The listing builds one solid part. Answer for the finished solid, in the listing's coordinates (mm). Give positions to 0.01 mm unless a question says otherwise; leave off trailing zeros. Loops run counter-clockwise (first coordinate to the right, second up) from the corner with the lowest first, then second, coordinate; pieces in that order, holes last. Notation, with made-up numbers: (8, -4) - (62, -4) arc R29 ccw to (62, 23) - close; hole circle Ø7 at (-11, -35). An arc over 180 degrees is marked (long way). Write each question's results on one line, items separated by ' | '.
from build123d import *

# Parameters (mm, degrees)
SKETCH4_R           = 4.5
BOSS_EXTRUDE1_DEPTH = 4.5
SKETCH5_OUTSIDE_W   = 56.268
SKETCH5_OUTSIDE_H   = 53.856
SKETCH5_OUTSIDE_R   = 7.794228634
CUT_EXTRUDE1_DEPTH  = 9
CUT_EXTRUDE1_TAPER  = 60


with BuildPart() as part:
    # Sketch4 → Boss-Extrude1 (new body, symmetric)
    with BuildSketch(Plane.XY):
        Polygon((4.5, 7.794228634), (-4.5, 7.794228634), (-9, 0), (-4.5, -7.794228634), (4.5, -7.794228634), (9, 0), align=None)
        Circle(SKETCH4_R, mode=Mode.SUBTRACT)
    extrude(amount=BOSS_EXTRUDE1_DEPTH, both=True)

    # Sketch5 outside → Cut-Extrude1 (cut)
    with BuildSketch(Plane.XY.offset(4.5)):
        Rectangle(SKETCH5_OUTSIDE_W, SKETCH5_OUTSIDE_H)
        Circle(SKETCH5_OUTSIDE_R, mode=Mode.SUBTRACT)
    cut_extrude1 = extrude(amount=-CUT_EXTRUDE1_DEPTH, taper=CUT_EXTRUDE1_TAPER, mode=Mode.SUBTRACT)

    # Mirror1: Cut-Extrude1 across plane
    add(cut_extrude1.mirror(Plane.XY), mode=Mode.SUBTRACT)


solid = part.part
Item 1: A flat-ended cylindrical pin translates along its axis: P1, Ø1.5, axis at y = -1.5, z = 2.5, coming from the +X side. Find the tip coordinate at first contact, or state that the pin passes through.
Values found:
P1: stops at x = 8.57
Item 2: Find the intervals of material crossed by line 1 along Y through (x, z) = (0, 1); line 2 along X through (y, z) = (2.75, -0.25); line 3 along X through (y, z) = (-3.75, 0), in increasing order. Write a range as [from, to].
Values found:
line 1: y = [-7.79, -4.5], [4.5, 7.79] | line 2: x = [-7.41, -3.56], [3.56, 7.41] | line 3: x = [-6.83, -2.49], [2.49, 6.83]
Item 3: A cutting plane is placed at A-A, the plane z = -2.5. Determine the outline of the cut face in (x, y).
Values found:
outline: (-9, 0) - (-4.5, -7.79) - (4.5, -7.79) - (9, 0) - (4.5, 7.79) - (-4.5, 7.79) - close; hole circle Ø9 at (0, 0)
Item 4: For a pull along X with two mould halves and no side action, classify faces 1 (the face through (6.781, 3.843, 0.063)), 2 (the face through (-0.59, 4.46, -0.06)), 3 (the face through (-8.09, -0.02, 4.33)) as released by +X, released by -X, zero draft, split by the parting line, or undercut.
Values found:
face 1: released by +X | face 2: undercut | face 3: released by -X
